Geometry check sheet. Reference: drawing and pictorial views, mm from the part's lowest x, y, z. Round coordinates to 2 decimals unless told otherwise and drop trailing zeros. Loops run counter-clockwise (first coordinate to the right, second up) from the corner with the lowest first, then second, coordinate; pieces in that order, holes last. Notation, with made-up numbers: (50.25, 30.5) - (78.25, 30.5) arc R18 ccw to (78.25, 44.5) - close; hole circle Ø11 at (-13.5, -10.5). An arc over 180 degrees is marked (long way). Return JSON: item names as keys, results as strings.
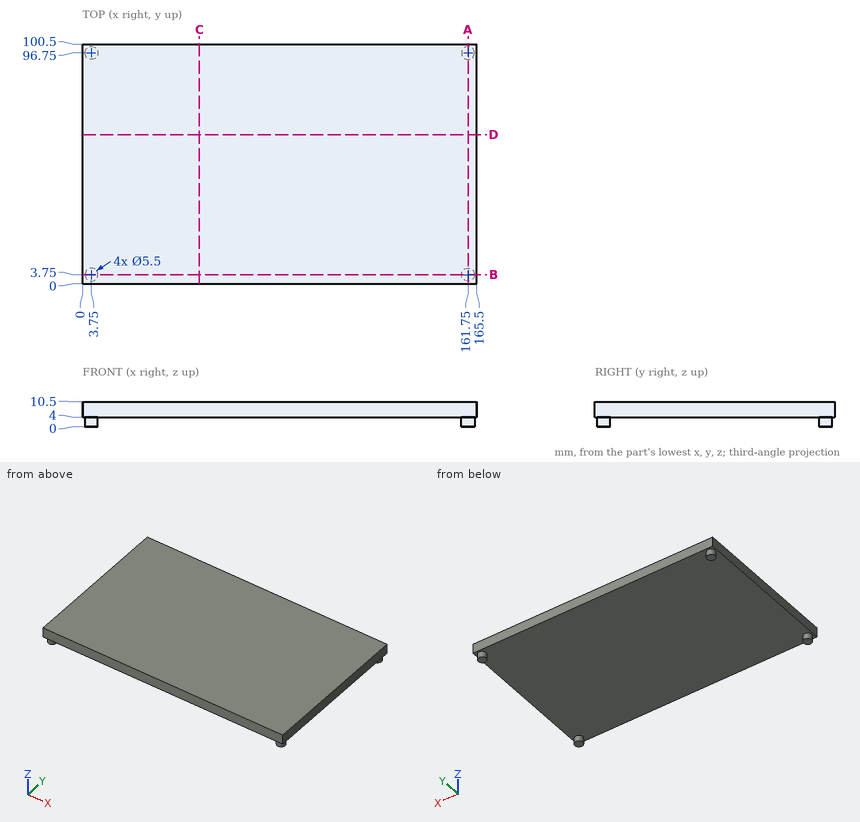
Q1. Depth check by flat-ended pin: P1, Ø8, axis at x = 31.5, y = 75.5, coming from the -Z side. Enter the tip coordinate at first touch or a pass-through.
Answer key:
{"P1": "stops at z = 4"}
Q2. Sectioned sample at A-A (x = 161.75). Enter the section's corners in (y, z), plus the area to 3 significant figures.
Answer key:
{"outline": "(0, 4) - (1, 4) - (1, 0) - (6.5, 0) - (6.5, 4) - (94, 4) - (94, 0) - (99.5, 0) - (99.5, 4) - (100.5, 4) - (100.5, 10.5) - (0, 10.5) - close", "area": "697 mm²"}
Q3. Sectioned sample at C-C (x = 49). Enter the section's corners in (y, z).
Answer key:
{"outline": "(0, 4) - (100.5, 4) - (100.5, 10.5) - (0, 10.5) - close"}
Q4. Sectioned sample at D-D (y = 62.5). Enter the section's corners in (x, z).
Answer key:
{"outline": "(0, 4) - (165.5, 4) - (165.5, 10.5) - (0, 10.5) - close"}
Q5. Scan lines: probe 1 along Z at (x, y) = (124, 93.5); probe 2 along X at (y, z) = (95.5, 2). Record each from-to range of solid material in increasing order. Write a range as [from, to].
Answer key:
{"probe 1": "z = [4, 10.5]", "probe 2": "x = [1.3, 6.2], [159.3, 164.2]"}
Q6. Sectioned sample at B-B (y = 3.75). Enter the section's corners in (x, z), plus the area to 3 significant figures.
Answer key:
{"outline": "(0, 4) - (1, 4) - (1, 0) - (6.5, 0) - (6.5, 4) - (159, 4) - (159, 0) - (164.5, 0) - (164.5, 4) - (165.5, 4) - (165.5, 10.5) - (0, 10.5) - close", "area": "1,120 mm²"}
